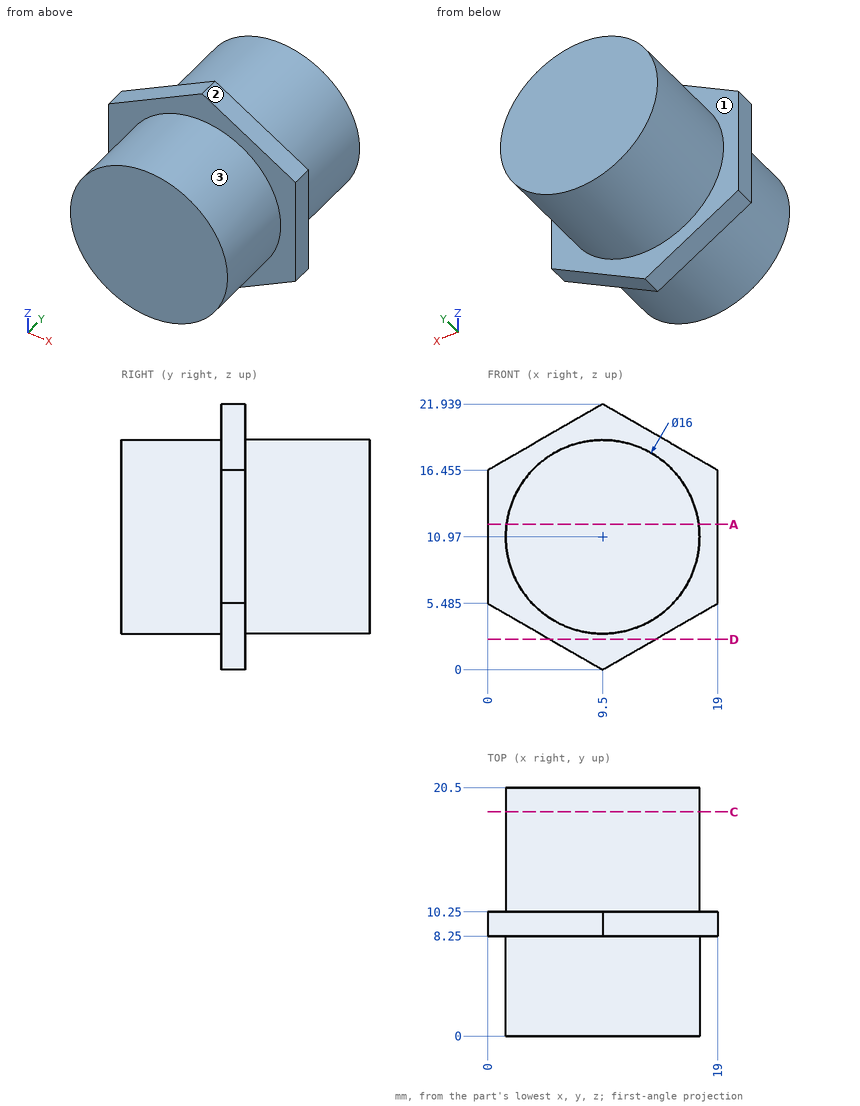
Study the drawing (mm; zero at the part's minimum x, y, z) and answer. A direction names the side the tool comes from. Give positions to 0.01 mm unless a question says otherwise; leave off trailing zeros. Write each loop counter-clockwise with the first axis right and the second up, starting at its lowest first coordinate (ties: lowest second). Pieces come first, ordered by that corner, then holes. Notation, with made-up numbers: (-33.75, -4.75) -> (-19.75, -4.75) arc R13 ccw to (-19.75, 6.25) -> close; hole circle Ø2 at (-39, -16.5). An arc over 180 degrees is marked (long way). Write item = value, one per line. Start each with the question number.
1) Straight lines are drawn through the part: line 1 along X through (y, z) = (18.5, 11.25) (1 decimal); line 2 along Y through (x, z) = (12.5, 19.25); line 3 along Z through (x, y) = (15.25, 12.75) (1 decimal). For each, find the intervals that lie inside material, in ascending order.
2) The part is cut by section A-A, the plane z = 12. Determine the outline of the cut face in (x, y).
3) The part is cut by section C-C, the plane y = 18.5. Determine the outline of the cut face in (x, z), and give its area (3 significant figures).
4) Which of the six approach directions +Z, -Z, +X, -X, +Y, -Y give full straight-line access (tool end or side, diameter ignored) to the marked faces 1, 2 and 3?
5) Each of these flat-tipped pins is pushed along its axis until it touches: pin 1 (10 mm diameter, centred on x = 3.5, y = 12, fed in from -Z); pin 2 (1 mm diameter, centred on y = 13.5, z = 6, fed in from +X) (1 decimal); pin 3 (3 mm diameter, centred on y = 2.5, z = 16.5, fed in from -X). Where does it stop, or does it pass through?
6) The part is cut by section D-D, the plane z = 2.5. Determine the outline of the cut face in (x, y).
Solutions:
q1.line_1 = 1.5 to 17.5
q1.line_2 = 8.25 to 10.25
q1.line_3 = 5.4 to 16.5
q2.outline = (0, 8.25) -> (1.57, 8.25) -> (1.57, 0) -> (17.43, 0) -> (17.43, 8.25) -> (19, 8.25) -> (19, 10.25) -> (17.43, 10.25) -> (17.43, 20.5) -> (1.57, 20.5) -> (1.57, 10.25) -> (0, 10.25) -> close
q3.outline = circle Ø16 at (9.5, 10.97)
q3.area = 201 mm²
q4.face_1 = +Y
q4.face_2 = +Z, +X, +Y, -Y
q4.face_3 = -Y
q5.pin_1 = 0.76
q5.pin_2 = 16.1
q5.pin_3 = 2.59
q6.outline = (5.17, 8.25) -> (13.83, 8.25) -> (13.83, 10.25) -> (5.17, 10.25) -> close
